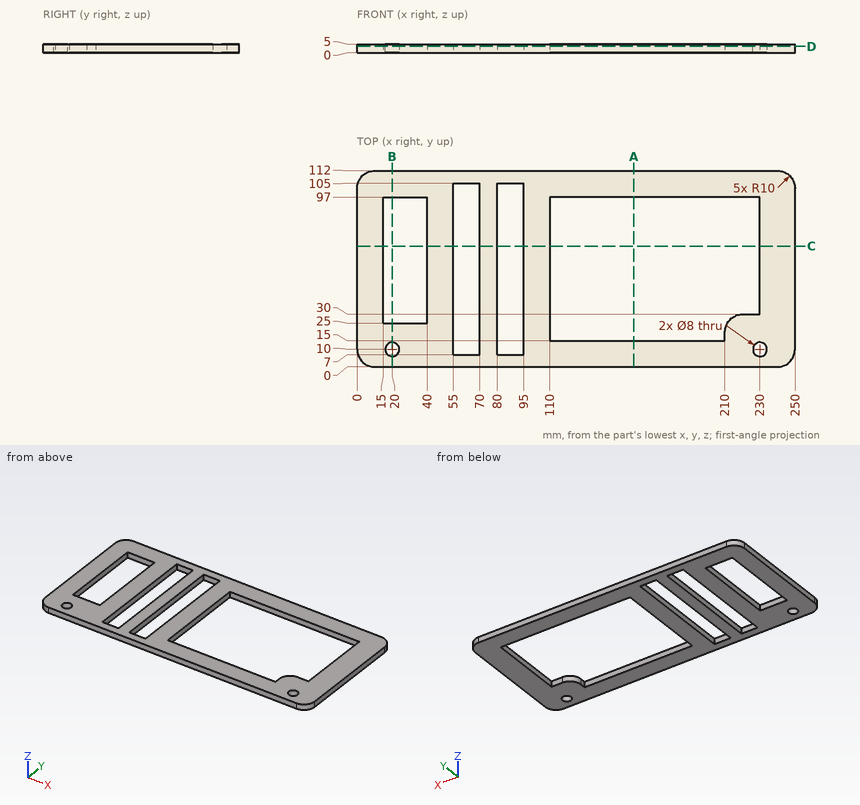
The figure shows three views and two pictorial views of one solid part (mm, origin at its lowest corner). Answer the questions. Round coordinates to 2 decimals unless told otherwise and drop trailing zeros. Write each loop counter-clockwise with the first axis right and the second up, starting at its lowest first coordinate (ties: lowest second). Pieces come first, ordered by that corner, then holes. Notation, with made-up numbers: (-33, 17) -> (-2, 17) arc R17 cw to (-2, 38) -> close; hole circle Ø1 at (40.25, 54.5). An arc over 180 degrees is marked (long way). Answer as a JSON object with one key per item and string values. Group by question number.
Q1. Section D-D (z = 3.65) is taken. Count the separate pieces of the cut face and the enclosed holes in it, plus the area to 3 significant figures.
Q2. Straight lines are drawn through the part: line 1 along X through (y, z) = (40.5, 2.2); line 2 along Y through (x, z) = (20, 3.5); line 3 along X through (y, z) = (100.5, 2.7). For each, find the intervals that lie inside material, in ascending order.
Q3. Section C-C (y = 69) is taken. Write down the section's boundary in (x, z), plus the area to 3 significant figures.
Q4. Section A-A (x = 158) is taken. Write down the section's boundary in (y, z).
Q5. Section B-B (x = 20) is taken. Write down the section's boundary in (y, z).
Check values:
{
 "1": {"separate pieces": "1", "enclosed holes": "6", "area": "13,500 mm^2"},
 "2": {"line 1": "0 to 15, 40 to 55, 70 to 80, 95 to 110, 230 to 250", "line 2": "0 to 6, 14 to 25, 97 to 112", "line 3": "0 to 55, 70 to 80, 95 to 250"},
 "3": {"outline": "(0, 0) -> (15, 0) -> (15, 5) -> (0, 5) -> close; (40, 0) -> (55, 0) -> (55, 5) -> (40, 5) -> close; (70, 0) -> (80, 0) -> (80, 5) -> (70, 5) -> close; (95, 0) -> (110, 0) -> (110, 5) -> (95, 5) -> close; (230, 0) -> (250, 0) -> (250, 5) -> (230, 5) -> close", "area": "375 mm^2"},
 "4": {"outline": "(0, 0) -> (15, 0) -> (15, 5) -> (0, 5) -> close; (97, 0) -> (112, 0) -> (112, 5) -> (97, 5) -> close"},
 "5": {"outline": "(0, 0) -> (6, 0) -> (6, 5) -> (0, 5) -> close; (14, 0) -> (25, 0) -> (25, 5) -> (14, 5) -> close; (97, 0) -> (112, 0) -> (112, 5) -> (97, 5) -> close"}
}
